Source: three-view drawing plus pictorial views. Frame: mm from the lowest corner of the part. A direction names the side the tool comes from. Give positions to 0.01 mm unless a question says otherwise; leave off trailing zeros. Loops run counter-clockwise (first coordinate to the right, second up) from the corner with the lowest first, then second, coordinate; pieces in that order, holes last. Notation, with made-up numbers: (44.5, 38.5) -> (65.5, 38.5) arc R23 cw to (65.5, 75.5) -> close; hole circle Ø7 at (-15, -7.5). An arc over 180 degrees is marked (long way). Answer in a Markdown table with one row per item. Add a question column.
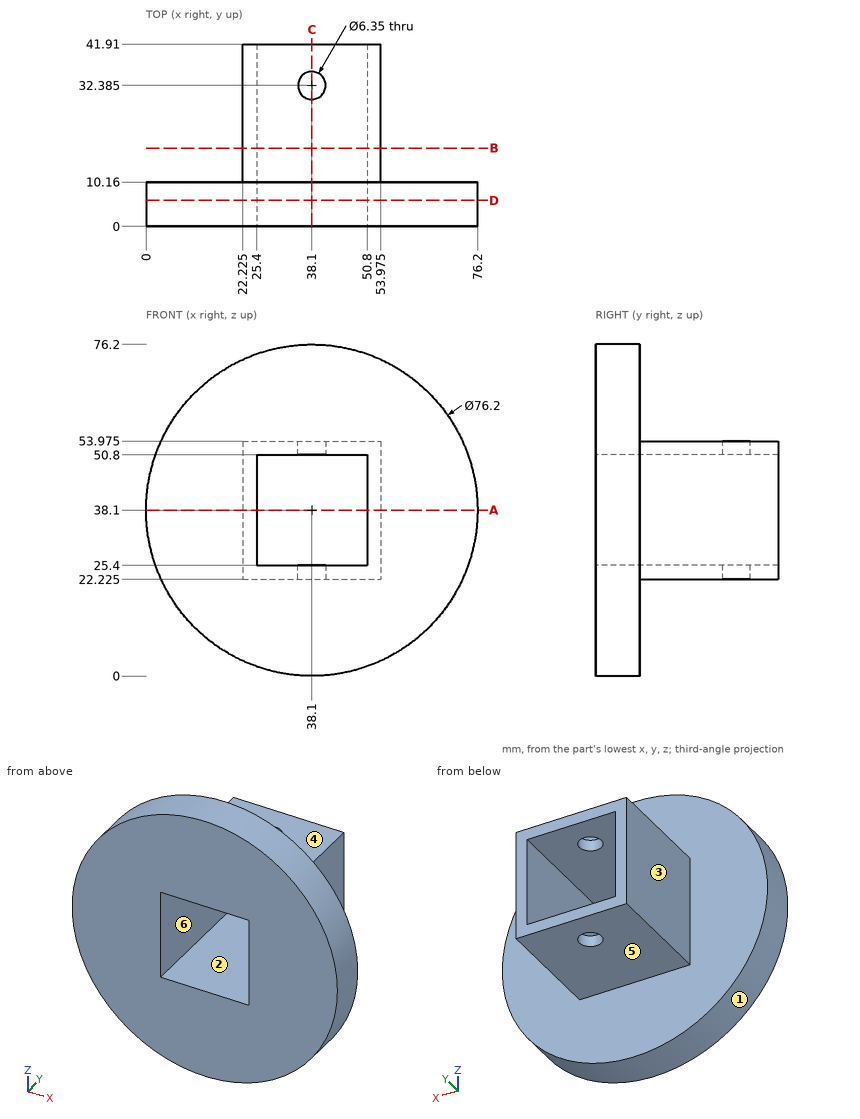
(1) Draft query along Z for the marked faces 1, 2 and 3. Return one class per face: +Z half, -Z half, draft (parallel to the pull), parting line (faces both ways), or undercut.
(2) Cut plane B-B on y = 18. Return the cut outline in (x, z) (3 decimals).
(3) Material intervals for line 1 along Y through (x, z) = (38, 52); line 2 along X through (y, z) = (39.5, 49) (3 decimals), sorted ascending. Write a range as from..to.
(4) Cut plane A-A on z = 38.1. Return the cut outline in (x, y) (3 decimals), then the cut area to 3 significant figures.
(5) Pin query (flat end, axial travel): pin 1 Ø4 at (x, z) = (39.5, 63.5) entering from +Y; pin 2 Ø20.5 at (y, z) = (31.5, 32.5) entering from -X (3 decimals); pin 3 Ø12 at (y, z) = (31, 27) entering from +X (3 decimals). Return the tip coordinate at first contact, or that it passes through.
(6) Cut plane D-D on y = 6. Return the cut outline in (x, z).
(7) Cut plane C-C on x = 38.1. Return the cut outline in (y, z) (3 decimals), then the cut area to 3 significant figures.
(8) Reachability of the marked faces 4, 5 and 6 from +Z, -Z, +X, -X, +Y, -Y: full face, straight path, thin tool, end or side. Return the list, or none.
Answer list:
| question | item | result |
|---|---|---|
| 1 | face 1 | parting line |
| 1 | face 2 | undercut |
| 1 | face 3 | draft |
| 2 | outline | (22.225, 22.225) -> (53.975, 22.225) -> (53.975, 53.975) -> (22.225, 53.975) -> close; hole (25.4, 25.4) -> (50.8, 25.4) -> (50.8, 50.8) -> (25.4, 50.8) -> close |
| 3 | line 1 | y = 0..29.21, 35.56..41.91 |
| 3 | line 2 | x = 22.225..25.4, 50.8..53.975 |
| 4 | outline | (0, 0) -> (25.4, 0) -> (25.4, 41.91) -> (22.225, 41.91) -> (22.225, 10.16) -> (0, 10.16) -> close; (50.8, 0) -> (76.2, 0) -> (76.2, 10.16) -> (53.975, 10.16) -> (53.975, 41.91) -> (50.8, 41.91) -> close |
| 4 | area | 718 mm² |
| 5 | pin 1 | stops at y = 10.16 |
| 5 | pin 2 | stops at x = 22.225 |
| 5 | pin 3 | stops at x = 53.975 |
| 6 | outline | circle Ø76.2 at (38.1, 38.1); hole (25.4, 25.4) -> (50.8, 25.4) -> (50.8, 50.8) -> (25.4, 50.8) -> close |
| 7 | outline | (0, 0) -> (10.16, 0) -> (10.16, 22.225) -> (29.21, 22.225) -> (29.21, 25.4) -> (0, 25.4) -> close; (0, 50.8) -> (29.21, 50.8) -> (29.21, 53.975) -> (10.16, 53.975) -> (10.16, 76.2) -> (0, 76.2) -> close; (35.56, 22.225) -> (41.91, 22.225) -> (41.91, 25.4) -> (35.56, 25.4) -> close; (35.56, 50.8) -> (41.91, 50.8) -> (41.91, 53.975) -> (35.56, 53.975) -> close |
| 7 | area | 677 mm² |
| 8 | face 4 | +Z, +X, -X, +Y |
| 8 | face 5 | -Z, +X, -X, +Y |
| 8 | face 6 | +Y, -Y |
